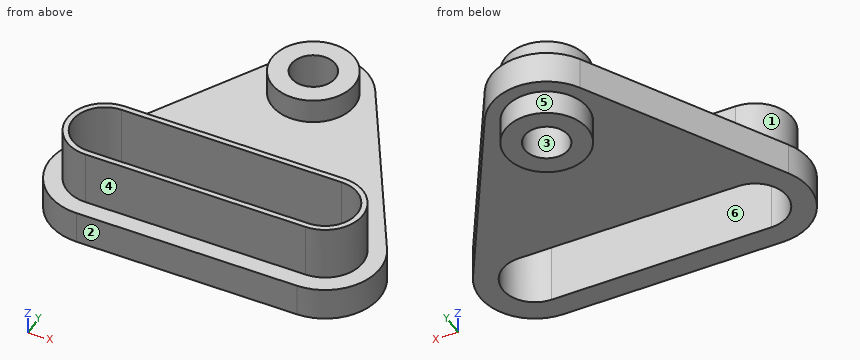
Autodesk Inventor part; units mm, degrees
ref_plane "YZ Plane" through (0, 0, 0) normal (1, 0, 0) x (0, 1, 0)
ref_plane "XZ Plane" through (0, 0, 0) normal (0, 1, 0) x (-1, 0, 0)
ref_plane "XY Plane" through (0, 0, 0) normal (0, 0, 1) x (1, 0, 0)
sketch "Sketch1" plane through (0, 0, 0) normal (0, 0, 1) x (1, 0, 0)
  arc A0 (8.6603, 39.641) -> (-8.6603, 39.641) centre (0, 34.641) ccw
  arc A1 (-28.6603, 5) -> (-20, -10) centre (-20, 0) ccw
  arc A2 (20, -10) -> (28.6603, 5) centre (20, 0) ccw
  line L0 (-8.6603, 39.641) -> (-28.6603, 5)
  line L1 (-20, -10) -> (20, -10)
  line L2 (28.6603, 5) -> (8.6603, 39.641)
  circle A3 centre (0, 34.641) radius 7.5
  line L3 (0, 56.0692) -> (0, -23.9282)
  line L4 (-46.1865, 0) -> (46.1865, 0)
  circle A4 centre (0, 34.641) radius 4
  point P0 (0, 0)
  dimension "d0" = 10
  dimension "d1" = 40
  dimension "d2" = 15
  dimension "d7" = 8
extrude "Extrusion1" add sketch "Sketch1" along normal mid plane 6
extrude "Extrusion2" add sketch "Sketch1" along normal mid plane 15 contours L3 A4 A3 | A3 L3 A4 | A4 L3 | L3 A4
extrude "Extrusion3" cut sketch "Sketch1" along normal through all both and the other way through all contours A4 L3 | L3 A4
sketch "Sketch2" plane through (0, 0, 3) normal (0, 0, 1) x (1, 0, 0)
  circle A0 centre (0, 34.641) radius 7.5
  line L0 (-8.6603, 39.641) -> (-28.6603, 5)
  arc A1 (-28.6603, 5) -> (-20, -10) centre (-20, 0) ccw
  line L1 (-20, -10) -> (20, -10)
  arc A2 (20, -10) -> (28.6603, 5) centre (20, 0) ccw
  line L2 (28.6603, 5) -> (8.6603, 39.641)
  arc A3 (-20, 6.85) -> (-20, -6.85) centre (-20, 0) ccw
  line L3 (-20, -6.85) -> (20, -6.85)
  arc A4 (20, -6.85) -> (20, 6.85) centre (20, 0) ccw
  line L4 (-20, 6.85) -> (20, 6.85)
  arc A5 (8.6603, 39.641) -> (-8.6603, 39.641) centre (0, 34.641) ccw
  point P0 (0, 0)
  dimension "d10" = 3.15
extrude "Extrusion4" add sketch "Sketch2" along normal blind 10 contours L4 A4 L3 A3
sketch "Sketch3" plane through (0, 0, 13) normal (0, 0, 1) x (1, 0, 0)
  line L0 (-20, -6.85) -> (20, -6.85)
  arc A0 (20, -6.85) -> (20, 6.85) centre (20, 0) ccw
  line L1 (20, 6.85) -> (-20, 6.85)
  arc A1 (-20, 6.85) -> (-20, -6.85) centre (-20, 0) ccw
  line L2 (20, -5.85) -> (-20, -5.85)
  arc A2 (-20, 5.85) -> (-20, -5.85) centre (-20, 0) ccw
  line L3 (-20, 5.85) -> (20, 5.85)
  arc A3 (20, -5.85) -> (20, 5.85) centre (20, 0) ccw
  point P0 (0, 0)
  dimension "d13" = 1
extrude "Extrusion5" cut sketch "Sketch3" against normal through all contours L2 A2 L3 A3
properties part number "Offset"
Design review of the part built by this model. Coordinates are the model's own, in mm. Face numbers are marked on the shaded views. A direction names the side the tool comes from. Round coordinates to 2 decimals unless told otherwise and drop trailing zeros. Write each loop counter-clockwise with the first axis right and the second up, starting at its lowest first coordinate (ties: lowest second). Pieces come first, ordered by that corner, then holes. Notation, with made-up numbers: (-15.5, 11) -> (13.5, 11) arc R26 ccw to (13.5, 34) -> close; hole circle Ø4 at (36, 44). An arc over 180 degrees is marked (long way). Answer in a Markdown table with one row per item.
Q1. To check wall thickness, follow L1, parallel to Y at x = 0, z = 2; L2, parallel to Y at x = -19, z = 11.5; L3, parallel to Y at x = -20, z = -1.25. State the ranges of each line that lie inside material, in increasing order. Write a range as [from, to].
The answers:
| item | result |
|---|---|
| L1 | [-10, -5.85], [5.85, 30.64], [38.64, 44.64] |
| L2 | [-6.85, -5.85], [5.85, 6.85] |
| L3 | [-10, -5.85], [5.85, 20] |
Q2. Take a section at D-D, the plane z = 8.75. State the section outline as (x, y) points.
The answers:
| item | result |
|---|---|
| outline | (-20, -6.85) -> (20, -6.85) arc R6.85 ccw to (20, 6.85) -> (-20, 6.85) arc R6.85 ccw to start; hole (-20, -5.85) -> (20, -5.85) arc R5.85 ccw to (20, 5.85) -> (-20, 5.85) arc R5.85 ccw to start |
Q3. Clearance check with flat-ended pins moving along their axes: pin 1 Ø1.5 at (x, y) = (7, 19.5) entering from -Z; pin 2 Ø6 at (x, z) = (-24, 9) entering from -Y; pin 3 Ø3 at (x, z) = (-1.5, 10) entering from +Y. State where each tip first meets the part, or that it passes through.
The answers:
| item | result |
|---|---|
| pin 1 | z = -3 |
| pin 2 | y = -6.78 |
| pin 3 | y = 6.85 |
Q4. For the marked faces 4, 5 and 6, list the 3-axis set-ups (+Z, -Z, +X, -X, +Y, -Y) from which the entire face can be reached by the end or side of a thin tool; tool diameter is ignored.
The answers:
| item | result |
|---|---|
| face 4 | +Z, +X, -X, -Y |
| face 5 | -Z |
| face 6 | +Z, -Z |
Q5. Take a section at C-C, the plane z = 5. State the section outline as (x, y) points, then the cut area to 3 significant figures.
The answers:
| item | result |
|---|---|
| outline | (-20, -6.85) -> (20, -6.85) arc R6.85 ccw to (20, 6.85) -> (-20, 6.85) arc R6.85 ccw to start; circle Ø15 at (0, 34.64); hole (-20, -5.85) -> (20, -5.85) arc R5.85 ccw to (20, 5.85) -> (-20, 5.85) arc R5.85 ccw to start; hole circle Ø8 at (0, 34.64) |
| area | 246 mm² |
Q6. Draft analysis for pull direction Y (two halves, no side actions). For the marked faces 1, 2 and 3, state which applies: +Y half, -Y half, draft (parallel to the pull), parting line (faces both ways), or undercut.
The answers:
| item | result |
|---|---|
| face 1 | parting line |
| face 2 | -Y half |
| face 3 | undercut |
Q7. Take a section at B-B, the plane x = 0. State the section outline as (y, z) points.
The answers:
| item | result |
|---|---|
| outline | (-10, -3) -> (-5.85, -3) -> (-5.85, 13) -> (-6.85, 13) -> (-6.85, 3) -> (-10, 3) -> close; (5.85, -3) -> (27.14, -3) -> (27.14, -7.5) -> (30.64, -7.5) -> (30.64, 7.5) -> (27.14, 7.5) -> (27.14, 3) -> (6.85, 3) -> (6.85, 13) -> (5.85, 13) -> close; (38.64, -7.5) -> (42.14, -7.5) -> (42.14, -3) -> (44.64, -3) -> (44.64, 3) -> (42.14, 3) -> (42.14, 7.5) -> (38.64, 7.5) -> close |
Q8. Take a section at A-A, the plane y = 0. State the section outline as (x, z) points, then the cut area to 3 significant figures.
The answers:
| item | result |
|---|---|
| outline | (-30, -3) -> (-25.85, -3) -> (-25.85, 13) -> (-26.85, 13) -> (-26.85, 3) -> (-30, 3) -> close; (25.85, -3) -> (30, -3) -> (30, 3) -> (26.85, 3) -> (26.85, 13) -> (25.85, 13) -> close |
| area | 69.8 mm² |
